```python
from build123d import *

# Parameters (mm, degrees)
EXTRUDE_THIN1_DEPTH = 12.7
SKETCH2_R           = 2.4892
CUT_EXTRUDE1_DEPTH  = 4.175


with BuildPart() as part:
    # Sketch1 → Extrude-Thin1 (new body, symmetric)
    with BuildSketch(Plane.XY):
        Polygon((0, 25.4), (0, 0), (25.4, 0), (25.4, 3.175), (3.175, 3.175), (3.175, 25.4), align=None)
    extrude(amount=EXTRUDE_THIN1_DEPTH, both=True)

    # Sketch2 → Cut-Extrude1 (cut, through all)
    with BuildSketch(Plane(origin=(0, 3.175, 0), x_dir=(1, 0, 0), z_dir=(0, 1, 0))):
        with Locations((12.7, 0)):
            Circle(SKETCH2_R)
    cut_extrude1 = extrude(amount=-CUT_EXTRUDE1_DEPTH, mode=Mode.SUBTRACT)

    # Mirror1: Cut-Extrude1 across plane
    add(cut_extrude1.mirror(Plane(origin=(0, 0, 0), x_dir=(0, 0, 1), z_dir=(0.707106781, -0.707106781, 0))), mode=Mode.SUBTRACT)


solid = part.part
```
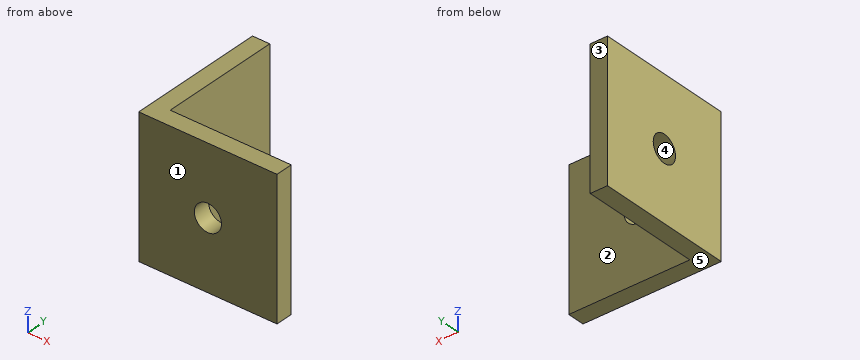
Geometry check sheet. Reference: the model listing, model coordinates, mm. Face numbers are marked on the shaded views. A direction names the side the tool comes from. Coordinates: 2 decimals unless noted, no trailing zeros. Write each loop counter-clockwise with the first axis right and the second up, starting at its lowest first coordinate (ties: lowest second). Pieces come first, ordered by that corner, then holes. Notation, with made-up numbers: M -5,62 L 0,62 A24 cw 0,76 Z; hole C 23.5,69.5 d6. An arc over 180 degrees is marked long. One line per item, written item: value. Start each with the question number.
(1) Scan lines: line 1 along Z through (x, y) = (2.2, 12.7); line 2 along Y through (x, z) = (1.45, 0). Record each from-to range of solid material in increasing order. Write a range as [from, to].
(2) Sectioned sample at D-D, the plane z = 6.5. Enter the section's corners in (x, y) (3 decimals).
(3) Depth check by flat-ended pin: pin 1 (1.5 mm diameter, centred on y = 11.5, z = 8.5, fed in from +X) (3 decimals); pin 2 (12 mm diameter, centred on x = 16.5, z = 4.5, fed in from +Y) (3 decimals). Enter the tip coordinate at first touch or a pass-through.
(4) Release check for a two-part mould opening along Y. For the marked faces 3, 4 and 5 record: released by +Y, released by -Y, zero draft, split by the parting line, or undercut.
(5) Sectioned sample at C-C, the plane z = 0. Enter the section's corners in (x, y) (3 decimals).
(6) Sectioned sample at A-A, the plane x = 12.7. Enter the section's corners in (y, z) (3 decimals), and give its area (3 significant figures).
(7) Tool access check on the marked faces 1 and 2. Record the directions out of +Z, -Z, +X, -X, +Y, -Y that give a thin tool (end or side, any length) a straight path to the whole face; none if there is none.
Filled sheet:
1. line 1: [-12.7, -2.49], [2.49, 12.7]
1. line 2: [0, 10.21], [15.19, 25.4]
2. outline: M 0,0 L 25.4,0 L 25.4,3.175 L 3.175,3.175 L 3.175,25.4 L 0,25.4 Z
3. pin 1: x = 3.175
3. pin 2: y = 3.175
4. face 3: released by +Y
4. face 4: undercut
4. face 5: zero draft
5. outline: M 0,0 L 10.211,0 L 10.211,3.175 L 3.175,3.175 L 3.175,10.211 L 0,10.211 Z; M 0,15.189 L 3.175,15.189 L 3.175,25.4 L 0,25.4 Z; M 15.189,0 L 25.4,0 L 25.4,3.175 L 15.189,3.175 Z
6. outline: M 0,-12.7 L 3.175,-12.7 L 3.175,-2.489 L 0,-2.489 Z; M 0,2.489 L 3.175,2.489 L 3.175,12.7 L 0,12.7 Z
6. area: 64.8 mm²
7. face 1: +Z, -Z, +X, -X, -Y
7. face 2: +Z, -Z, +X, +Y
